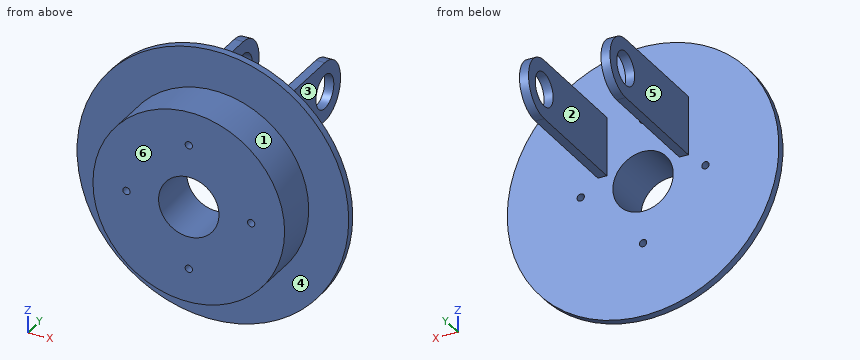
```python
from build123d import *

# Parameters (mm, degrees)
SKETCH_1_R          = 90
EXTRUDE_2_DEPTH     = 5
SKETCH_2_R          = 63.5
EXTRUDE_3_DEPTH     = 30
SKETCH_3_R          = 2.415
CUT_EXTRUDE_1_DEPTH = 36
SKETCH_4_W          = 6
SKETCH_4_H          = 39
EXTRUDE_4_DEPTH     = 78
EXTRUDE_START       = -6
EXTRUDE_5_DEPTH     = 6
EXTRUDE_6_DEPTH     = 6
SKETCH_8_R          = 11.1125
CUT_EXTRUDE_3_DEPTH = 121
SKETCH2_R           = 20
CUT_EXTRUDE1_DEPTH  = 36


with BuildPart() as part:
    # 草圖1 → 填料-伸長2 (new body)
    with BuildSketch(Plane(origin=(0, 0, 0), x_dir=(1, 0, 0), z_dir=(0, 1, 0))):
        Circle(SKETCH_1_R)
    extrude(amount=EXTRUDE_2_DEPTH)

    # 草圖2 → 填料-伸長3 (add)
    with BuildSketch(Plane.XZ):
        Circle(SKETCH_2_R)
    extrude(amount=EXTRUDE_3_DEPTH)

    # 草圖3 → 除料-伸長1 (cut, through all)
    with BuildSketch(Plane(origin=(0, 5, 0), x_dir=(1, 0, 0), z_dir=(0, 1, 0))):
        with Locations((0, 41.31)):
            Circle(SKETCH_3_R)
        with Locations((0, -41.31)):
            Circle(SKETCH_3_R)
        with Locations((-41.31, 0)):
            Circle(SKETCH_3_R)
        with Locations((41.31, 0)):
            Circle(SKETCH_3_R)
    extrude(amount=-CUT_EXTRUDE_1_DEPTH, mode=Mode.SUBTRACT)

    # 草圖4 → 填料-伸長4 (add)
    with BuildSketch(Plane(origin=(0, 5, 0), x_dir=(1, 0, 0), z_dir=(0, 1, 0))):
        with Locations((-27, -29.5)):
            Rectangle(SKETCH_4_W, SKETCH_4_H)
        with Locations((27, -29.5)):
            Rectangle(SKETCH_4_W, SKETCH_4_H)
    extrude(amount=EXTRUDE_4_DEPTH)

    # 草圖5 → 填料-伸長5 (add)
    with BuildSketch(Plane.ZY.offset(30).offset(EXTRUDE_START)):
        with BuildLine():
            Line((10, 83), (49, 83))
            ThreePointArc((49, 83), (29.5, 102.5), (10, 83))
        make_face()
    extrude(amount=EXTRUDE_5_DEPTH)

    # 草圖7 → 填料-伸長6 (add)
    with BuildSketch(Plane.ZY.offset(-24)):
        with BuildLine():
            Line((10, 83), (49, 83))
            ThreePointArc((49, 83), (29.5, 102.5), (10, 83))
        make_face()
    extrude(amount=-EXTRUDE_6_DEPTH)

    # 草圖8 → 除料-伸長3 (cut, through all)
    with BuildSketch(Plane.ZY.offset(30)):
        with Locations((29.5, 83)):
            Circle(SKETCH_8_R)
    extrude(amount=-CUT_EXTRUDE_3_DEPTH, mode=Mode.SUBTRACT)

    # Sketch2 → Cut-Extrude1 (cut, through all)
    with BuildSketch(Plane(origin=(0, 5, 0), x_dir=(1, 0, 0), z_dir=(0, 1, 0))):
        Circle(SKETCH2_R)
    extrude(amount=-CUT_EXTRUDE1_DEPTH, mode=Mode.SUBTRACT)


solid = part.part
```
Verification items for the finished model (mm, model axes). Face numbers are marked on the shaded views. A direction names the side the tool comes from. Give positions to 0.01 mm unless a question says otherwise; leave off trailing zeros. Write each loop counter-clockwise with the first axis right and the second up, starting at its lowest first coordinate (ties: lowest second). Pieces come first, ordered by that corner, then holes. Notation, with made-up numbers: (-36.5, 68) - (3.5, 68) arc R25 ccw to (3.5, 103) - close; hole circle Ø9 at (25.25, 13). An arc over 180 degrees is marked (long way). Put each result on its own line as item: value.
Q1. Section check B-B on x = 0. Record the cut outline in (y, z) (3 decimals).
Result:
outline: (-30, -63.5) - (0, -63.5) - (0, -90) - (5, -90) - (5, -43.725) - (-30, -43.725) - close; (-30, -38.895) - (5, -38.895) - (5, -20) - (-30, -20) - close; (-30, 20) - (5, 20) - (5, 38.895) - (-30, 38.895) - close; (-30, 43.725) - (5, 43.725) - (5, 90) - (0, 90) - (0, 63.5) - (-30, 63.5) - close
Q2. Section check D-D on z = -41.31. Record the cut outline in (x, y) (3 decimals).
Result:
outline: (-79.959, 0) - (-48.226, 0) - (-48.226, -30) - (-2.415, -30) - (-2.415, 5) - (-79.959, 5) - close; (2.415, -30) - (48.226, -30) - (48.226, 0) - (79.959, 0) - (79.959, 5) - (2.415, 5) - close
Q3. Scan lines: probe 1 along Z at (x, y) = (0, -14.5) (3 decimals); probe 2 along Y at (x, z) = (27, 29); probe 3 along X at (y, z) = (12, 30). Record each from-to range of solid material in increasing order. Write a range as from..to.
Result:
probe 1: -63.5..-43.725, -38.895..-20, 20..38.895, 43.725..63.5
probe 2: -30..71.9, 94.1..102.49
probe 3: -30..-24, 24..30
Q4. Section check C-C on y = 38.5. Record the cut outline in (x, z).
Result:
outline: (-30, 10) - (-24, 10) - (-24, 49) - (-30, 49) - close; (24, 10) - (30, 10) - (30, 49) - (24, 49) - close
Q5. Mould release check, pull along X, two halves, no side actions. Record for the marked faces 1, 2 and 3: released by +X, released by -X, zero draft, split by the parting line, or undercut.
Result:
face 1: split by the parting line
face 2: undercut
face 3: released by +X
Q6. Section check A-A on z = 0. Record the cut outline in (x, y) (3 decimals).
Result:
outline: (-90, 0) - (-63.5, 0) - (-63.5, -30) - (-43.725, -30) - (-43.725, 5) - (-90, 5) - close; (-38.895, -30) - (-20, -30) - (-20, 5) - (-38.895, 5) - close; (20, -30) - (38.895, -30) - (38.895, 5) - (20, 5) - close; (43.725, -30) - (63.5, -30) - (63.5, 0) - (90, 0) - (90, 5) - (43.725, 5) - close
Q7. Set-up check for the marked faces 4, 5 and 6: record each of +Z, -Z, +X, -X, +Y, -Y from which the full face is reachable in a straight line by a thin tool's end or side.
Result:
face 4: -Y
face 5: +Z, -Z, -X, +Y
face 6: +Z, -Z, +X, -X, -Y
Q8. Depth check by flat-ended pin: P1, Ø20, axis at y = 83, z = 29.5, coming from the -X side; P2, Ø6, axis at y = 58, z = 43.5, coming from the -X side; P3, Ø5, axis at x = 28, y = 63.5, coming from the +Z side; P4, Ø4, axis at x = -29, y = 37.5, coming from the -Z side. Enter the tip coordinate at first touch or a pass-through.
Result:
P1: through
P2: x = -30
P3: z = 49
P4: z = 10
